Autodesk Inventor part; units mm, degrees
ref_plane "YZ Plane" through (0, 0, 0) normal (1, 0, 0) x (0, 1, 0)
ref_plane "XZ Plane" through (0, 0, 0) normal (0, 1, 0) x (-1, 0, 0)
ref_plane "XY Plane" through (0, 0, 0) normal (0, 0, 1) x (1, 0, 0)
sketch "Sketch1" plane through (0, 0, 0) normal (1, 0, 0) x (0, 1, 0)
  line L0 (1.8986, 1.3831) -> (-40.1014, 1.3831)
  line L1 (-40.1014, 1.3831) -> (-40.1014, -42.3731)
  line L2 (-40.1014, -42.3731) -> (1.8986, -42.3731)
  line L3 (1.8986, -42.3731) -> (1.8986, 1.3831)
  point P0 (0, 0)
  dimension "d0" = 42
extrude "Extrusion1" add sketch "Sketch1" along normal blind 100
sketch "Sketch3" plane through (0, 0, 0) normal (-1, 0, 0) x (0, 0, 1)
  point P0 (0, 0)
sketch "Sketch8" plane through (0, 0, 0) normal (-1, 0, 0) x (0, 0, 1)
  point P0 (0, 0)
  point P1 (-20.6894, -17.7504)
hole "Hole4" at (0, -17.7504, -20.6894) direction (1, 0, 0) diameter 15.875 end through all
sketch "Sketch9" plane through (0, -40.1014, 1.3831) normal (0, 0, 1) x (1, 0, 0)
  line L0 (0, 42) -> (100, 42)
  line L1 (0, 0) -> (100, 0)
  line L2 (1.351, 42) -> (99.1356, 42)
  line L3 (99.1356, 42) -> (99.1356, 0)
  line L4 (99.1356, 0) -> (1.351, 0)
  line L5 (1.351, 0) -> (1.351, 42)
  point P0 (0, 40.1014)
  point P1 (1.351, 0)
extrude "Extrusion4" cut sketch "Sketch9" against normal blind 42
sketch "Sketch10" plane through (1.351, -40.1014, 1.3831) normal (1, 0, 0) x (0, 0, -1)
  line L0 (0, 42) -> (42, 42)
  line L1 (43.7562, 0) -> (43.7562, 42)
  line L2 (0, 42) -> (43.7562, 42)
  line L3 (43.7562, 42) -> (43.7562, 0)
  line L4 (43.7562, 0) -> (0, 0)
  line L5 (0, 0) -> (0, 42)
  point P0 (1.3831, 40.1014)
extrude "Extrusion5" cut sketch "Sketch10" against normal blind 25.4
sketch "Sketch11" plane through (0, -40.1014, -40.6169) normal (0, 0, 1) x (1, 0, 0)
  point P0 (0, 40.1014)
  point P1 (12.91, 21.6985)
hole "Hole5" at (12.91, -18.403, -40.6169) direction (0, 0, -1) diameter 5 end through all
sketch "Sketch12" plane through (100, 0, 0) normal (1, 0, 0) x (0, 0, -1)
  line L0 (42.3731, 1.8986) -> (-1.3831, 1.8986)
  line L1 (-1.3831, 1.8986) -> (42.3731, 1.8986)
  line L2 (42.3731, 1.8986) -> (42.3731, -40.1014)
  line L3 (42.3731, -40.1014) -> (-1.3831, -40.1014)
  line L4 (-1.3831, -40.1014) -> (-1.3831, 1.8986)
  point P0 (0, 0)
extrude "Extrusion6" add sketch "Sketch12" along normal blind 50.8
sketch "Sketch13" plane through (99.1356, -40.1014, 1.3831) normal (-1, 0, 0) x (0, 0, 1)
  line L0 (-42, 42) -> (0, 42)
  line L1 (0, 42) -> (0, 0)
  line L2 (-42, 42) -> (0, 42)
  line L3 (0, 42) -> (0, 0)
  line L4 (0, 0) -> (-42, 0)
  line L5 (-42, 0) -> (-42, 42)
  point P0 (-1.3831, 40.1014)
sketch "Sketch14" plane through (100, -17.7504, -20.6894) normal (-1, 0, 0) x (0, 0, 1)
  point P0 (20.6894, 17.7504)
  point P1 (-0.1562, -0.422)
hole "Hole6" at (100, -18.1724, -20.8455) direction (1, 0, 0) diameter 15.875 end through all
extrude "Extrusion7" cut sketch "Sketch13" against normal blind 48.26
sketch "Sketch15" plane through (0, -40.1014, -40.6169) normal (0, 0, 1) x (1, 0, 0)
  point P0 (0, 40.1014)
properties part number "clamp 2 pipe"
Geometry: final body of the model. Coordinates: model frame, mm. A direction names the side the tool comes from. Round coordinates to 2 decimals unless told otherwise and drop trailing zeros. Loops run counter-clockwise (first coordinate to the right, second up) from the corner with the lowest first, then second, coordinate; pieces in that order, holes last.
Q1. Material intervals for L1, parallel to Y at x = 12.91, z = -41.75; L2, parallel to Z at x = 92, y = -2.5; L3, parallel to X at y = -4.5, z = -26, sorted ascending.
Q2. Section D-D on x = 84. Return loops of the section in (y, z), plus the area to 3 significant figures.
Q3. Section C-C on y = -6.5. Return loops of the section in (x, z), plus the area to 3 significant figures.
Q4. Section B-B on z = -18. Return loops of the section in (x, y), plus the area to 3 significant figures.
Q5. Pin query (flat end, axial travel): P1, Ø3, axis at x = 12.91, y = -18.403, coming from the -Z side; P2, Ø12.5, axis at y = -26, z = -28, coming from the -X side; P3, Ø1, axis at x = 102.5, y = -35, coming from the +Z side. Return the tip coordinate at first contact, or that it passes through.
Q6. Access query for faces 4 (the flat face through (147.396, -19, -29)), 5 (the flat face through (109, -40.101, -42)). Directions: +Z, -Z, +X, -X, +Y, -Y. A direction counts if a zero-diameter tool reaches every point of the face in a straight line with its end or side. Return the directions, or none.
Q7. Section A-A on x = 12.91. Return loops of the section in (y, z).
Q8. Pull-direction query (Y, two-part tool) for faces 1 (the flat face through (150.8, -9, -20)), 2 (the flat face through (109, 1.899, -42)), 3 (the cylindrical face through (11.22, -16.56, -41.51)); classes: released by +Y, released by -Y, zero draft, split by the parting line, or undercut.
Evaluation:
1. L1: y = -40.1 to -20.9, -15.9 to 1.9
1. L2: z = -42.37 to -40.62
1. L3: x = 147.4 to 150.8
2. outline: (-40.1, -42.37) - (1.9, -42.37) - (1.9, -40.62) - (-40.1, -40.62) - close
2. area: 73.8 mm2
3. outline: (1.35, -42.37) - (150.8, -42.37) - (150.8, 1.38) - (147.4, 1.38) - (147.4, -40.62) - (1.35, -40.62) - close
3. area: 405 mm2
4. outline: (147.4, -40.1) - (150.8, -40.1) - (150.8, -25.58) - (147.4, -25.58) - close; (147.4, -10.76) - (150.8, -10.76) - (150.8, 1.9) - (147.4, 1.9) - close
4. area: 92.5 mm2
5. P1: passes through
5. P2: stops at x = 147.4
5. P3: stops at z = -40.62
6. face 4: +Z, -X, +Y, -Y
6. face 5: +Z, -Z, +X, -X, -Y
7. outline: (-40.1, -42.37) - (-20.9, -42.37) - (-20.9, -40.62) - (-40.1, -40.62) - close; (-15.9, -42.37) - (1.9, -42.37) - (1.9, -40.62) - (-15.9, -40.62) - close
8. face 1: zero draft
8. face 2: released by +Y
8. face 3: undercut
